Could you check a few things on this model? Use its own coordinates, in mm. A direction names the side the tool comes from. Give positions to 0.01 mm unless a question says otherwise; leave off trailing zeros. Write each loop counter-clockwise with the first axis right and the second up, starting at its lowest first coordinate (ties: lowest second). Pieces come first, ordered by that corner, then holes. Notation, with made-up numbers: M 64,5.25 L 89,5.25 A16 ccw 89,14.25 Z; hole C 53,72.25 d5. An arc over 180 degrees is marked long. Use one line per item in the form item = value.
from build123d import *

# Parameters (mm, degrees)
SKETCH1_R                             = 6
SKETCH1_R_2                           = 1.5
DISPLAY_SCREW_PATTERN_DEPTH           = 3
DISPLAY_SCREW_PATTERN_2_DEPTH         = 3
DISPLAY_SCREW_PATTERN_3_DEPTH         = 3
DISPLAY_SCREW_PATTERN_4_DEPTH         = 3
DISPLAY_SCREW_PATTERN_5_DEPTH         = 3
SKETCH2_W                             = 311.1
SKETCH2_H                             = 132.6
SKETCH2_R                             = 4
DISPLAY_BACKPLANE_DEPTH               = 3
BACKPLANE_WEIGHT_REDUCTION_DEPTH      = 203.770122306
BACKPLANE_WEIGHT_REDUCTION_DEPTH_BACK = 203.770122306
SKETCH4_W                             = 311.1
SKETCH4_H                             = 132.6
SKETCH4_W_2                           = 309.1
SKETCH4_H_2                           = 130.6
DISPLAY_OUTSIDE_CRADDLE_DEPTH         = 12
BOTTOM_RADIO_MOUNT_TABS_DEPTH         = 5
TOP_RADIO_MOUNT_TABS_DEPTH            = 5
TOP_RADIO_MOUNT_TABS_2_DEPTH          = 5
BOSS_EXTRUDE6_REACH                   = 208.065
BOSS_EXTRUDE7_REACH                   = 211.446
BOSS_EXTRUDE8_REACH                   = 213.846
BOSS_EXTRUDE9_REACH                   = 205.9
TAB_FILLETS_10MM_R                    = 10


with BuildPart() as part:
    # Sketch1 → Display screw pattern (new body)
    with BuildSketch(Plane.XY):
        Circle(SKETCH1_R)
        Circle(SKETCH1_R_2, mode=Mode.SUBTRACT)
    extrude(amount=DISPLAY_SCREW_PATTERN_DEPTH)



with BuildPart() as body_2:
    # Sketch1 → Display screw pattern 2 (new body)
    with BuildSketch(Plane.XY):
        with Locations((-106.24, 18.83)):
            Circle(SKETCH1_R)
        with Locations((-106.24, 18.83)):
            Circle(SKETCH1_R_2, mode=Mode.SUBTRACT)
    extrude(amount=DISPLAY_SCREW_PATTERN_2_DEPTH)


with BuildPart() as body_3:
    # Sketch1 → Display screw pattern 3 (new body)
    with BuildSketch(Plane.XY):
        with Locations((147.61, 18.83)):
            Circle(SKETCH1_R)
        with Locations((147.61, 18.83)):
            Circle(SKETCH1_R_2, mode=Mode.SUBTRACT)
    extrude(amount=DISPLAY_SCREW_PATTERN_3_DEPTH)


with BuildPart() as body_4:
    # Sketch1 → Display screw pattern 4 (new body)
    with BuildSketch(Plane.XY):
        with Locations((-121.24, -91.25)):
            Circle(SKETCH1_R)
        with Locations((-121.24, -91.25)):
            Circle(SKETCH1_R_2, mode=Mode.SUBTRACT)
    extrude(amount=DISPLAY_SCREW_PATTERN_4_DEPTH)


with BuildPart() as body_5:
    # Sketch1 → Display screw pattern 5 (new body)
    with BuildSketch(Plane.XY):
        with Locations((162.61, -91.25)):
            Circle(SKETCH1_R)
        with Locations((162.61, -91.25)):
            Circle(SKETCH1_R_2, mode=Mode.SUBTRACT)
    extrude(amount=DISPLAY_SCREW_PATTERN_5_DEPTH)


with BuildPart() as part_1:
    add(part.part)

    add(body_2.part)  # Display backplane merges body 2

    add(body_3.part)  # Display backplane merges body 3

    add(body_4.part)  # Display backplane merges body 4

    add(body_5.part)  # Display backplane merges body 5
    # Sketch2 → Display backplane (add)
    with BuildSketch(Plane(origin=(0, 0, 0), x_dir=(-1, 0, 0), z_dir=(0, 0, -1))):
        with Locations((-20.21, -34.77)):
            Rectangle(SKETCH2_W, SKETCH2_H)
        with Locations((106.24, 18.83)):
            Circle(SKETCH2_R, mode=Mode.SUBTRACT)
        Circle(SKETCH2_R, mode=Mode.SUBTRACT)
        with Locations((121.24, -91.25)):
            Circle(SKETCH2_R, mode=Mode.SUBTRACT)
        with Locations((-147.61, 18.83)):
            Circle(SKETCH2_R, mode=Mode.SUBTRACT)
        with Locations((-162.61, -91.25)):
            Circle(SKETCH2_R, mode=Mode.SUBTRACT)
    extrude(amount=DISPLAY_BACKPLANE_DEPTH)

    # Sketch3 → Backplane weight reduction (cut, two sides: drawn at the far end of the back side and taken through both)
    with BuildSketch(Plane.XY.offset(-BACKPLANE_WEIGHT_REDUCTION_DEPTH_BACK)):
        with BuildLine():
            Line((162.61, -7.17), (162.61, -67.25))
            ThreePointArc((162.61, -67.25), (160.930502943, -72.797001962), (156.456153846, -76.480769231))
            ThreePointArc((156.456153846, -76.480769231), (151.296291501, -79.936291501), (147.840769231, -85.096153846))
            ThreePointArc((147.840769231, -85.096153846), (144.157001962, -89.570502943), (138.61, -91.25))
            Line((138.61, -91.25), (-97.24, -91.25))
            ThreePointArc((-97.24, -91.25), (-102.787001962, -89.570502943), (-106.470769231, -85.096153846))
            ThreePointArc((-106.470769231, -85.096153846), (-109.926291501, -79.936291501), (-115.086153846, -76.480769231))
            ThreePointArc((-115.086153846, -76.480769231), (-119.560502943, -72.797001962), (-121.24, -67.25))
            Line((-121.24, -67.25), (-121.24, -7.17))
            ThreePointArc((-121.24, -7.17), (-118.311067812, -0.098932188), (-111.24, 2.83))
            Line((-111.24, 2.83), (-106.24, 2.83))
            ThreePointArc((-106.24, 2.83), (-97.36479686, 5.517195291), (-91.470769231, 12.676153846))
            ThreePointArc((-91.470769231, 12.676153846), (-87.787001962, 17.150502943), (-82.24, 18.83))
            Line((-82.24, 18.83), (-21, 18.83))
            ThreePointArc((-21, 18.83), (-13.928932188, 15.901067812), (-11, 8.83))
            Line((-11, 8.83), (-11, 0))
            ThreePointArc((-11, 0), (0, -11), (11, 0))
            Line((11, 0), (11, 8.83))
            ThreePointArc((11, 8.83), (13.928932188, 15.901067812), (21, 18.83))
            Line((21, 18.83), (123.61, 18.83))
            ThreePointArc((123.61, 18.83), (129.157001962, 17.150502943), (132.840769231, 12.676153846))
            ThreePointArc((132.840769231, 12.676153846), (138.73479686, 5.517195291), (147.61, 2.83))
            Line((147.61, 2.83), (152.61, 2.83))
            ThreePointArc((152.61, 2.83), (159.681067812, -0.098932188), (162.61, -7.17))
        make_face()
    extrude(amount=BACKPLANE_WEIGHT_REDUCTION_DEPTH + BACKPLANE_WEIGHT_REDUCTION_DEPTH_BACK, mode=Mode.SUBTRACT)

    # Sketch4 → Display outside craddle (add)
    with BuildSketch(Plane(origin=(0, 0, -3), x_dir=(-1, 0, 0), z_dir=(0, 0, -1))):
        with Locations((-20.21, -34.77)):
            Rectangle(SKETCH4_W, SKETCH4_H)
        with Locations((-20.21, -34.77)):
            Rectangle(SKETCH4_W_2, SKETCH4_H_2, mode=Mode.SUBTRACT)
    extrude(amount=DISPLAY_OUTSIDE_CRADDLE_DEPTH)

    # Sketch9 → Boss-Extrude6 (add, up to next)
    with BuildSketch(Plane(origin=(0, -9.845, 0), x_dir=(1, 0, 0), z_dir=(0, 1, 0)), mode=Mode.PRIVATE) as boss_extrude6_sk1:
        Polygon((109.074247912, 3), (134.956152423, 3), (135.76, 0), (109.87809549, 0), align=None)
    boss_extrude6_tool1 = extrude(boss_extrude6_sk1.sketch, amount=BOSS_EXTRUDE6_REACH, mode=Mode.PRIVATE) - part_1.part
    # Sketch9 → Boss-Extrude6 (add, up to next)
    with BuildSketch(Plane(origin=(0, -9.845, 0), x_dir=(1, 0, 0), z_dir=(0, 1, 0)), mode=Mode.PRIVATE) as boss_extrude6_sk2:
        Polygon((-58.122855224, 3), (-32.240950714, 3), (-31.437103136, 0), (-57.319007646, 0), align=None)
    boss_extrude6_tool2 = extrude(boss_extrude6_sk2.sketch, amount=BOSS_EXTRUDE6_REACH, mode=Mode.PRIVATE) - part_1.part


with BuildPart() as body_2_2:
    # Sketch5 → Bottom radio mount tabs (new body)
    with BuildSketch(Plane(origin=(0, -72.095, 0), x_dir=(1, 0, 0), z_dir=(0, 1, 0))):
        with BuildLine():
            Line((134.956152423, 3), (147.909153247, -45.341257188))
            ThreePointArc((147.909153247, -45.341257188), (147.20985029, -50.652990504), (142.959405779, -53.914471288))
            Line((142.959405779, -53.914471288), (132.33422169, -56.761480784))
            ThreePointArc((132.33422169, -56.761480784), (127.022488374, -56.062177826), (123.76100759, -51.811733316))
            Line((123.76100759, -51.811733316), (109.074247912, 3))
            Line((109.074247912, 3), (134.956152423, 3))
        make_face()
    extrude(amount=BOTTOM_RADIO_MOUNT_TABS_DEPTH)


with BuildPart() as body_3_2:
    # Sketch7 → Top radio mount tabs (new body)
    with BuildSketch(Plane(origin=(0, -14.845, 0), x_dir=(1, 0, 0), z_dir=(0, 1, 0))):
        with BuildLine():
            Line((-32.240950714, 3), (-19.287949889, -45.341257188))
            ThreePointArc((-19.287949889, -45.341257188), (-19.987252846, -50.652990504), (-24.237697357, -53.914471288))
            Line((-24.237697357, -53.914471288), (-34.862881446, -56.761480784))
            ThreePointArc((-34.862881446, -56.761480784), (-40.174614762, -56.062177826), (-43.436095546, -51.811733316))
            Line((-43.436095546, -51.811733316), (-58.122855224, 3))
            Line((-58.122855224, 3), (-32.240950714, 3))
        make_face()
    extrude(amount=TOP_RADIO_MOUNT_TABS_DEPTH)


with BuildPart() as body_4_2:
    # Sketch7 → Top radio mount tabs 2 (new body)
    with BuildSketch(Plane(origin=(0, -14.845, 0), x_dir=(1, 0, 0), z_dir=(0, 1, 0))):
        with BuildLine():
            Line((132.33422169, -56.761480784), (142.959405779, -53.914471288))
            ThreePointArc((142.959405779, -53.914471288), (147.20985029, -50.652990504), (147.909153247, -45.341257188))
            Line((147.909153247, -45.341257188), (134.956152423, 3))
            Line((134.956152423, 3), (109.074247912, 3))
            Line((109.074247912, 3), (123.76100759, -51.811733316))
            ThreePointArc((123.76100759, -51.811733316), (127.022488374, -56.062177826), (132.33422169, -56.761480784))
        make_face()
    extrude(amount=TOP_RADIO_MOUNT_TABS_2_DEPTH)


with BuildPart() as part_2:
    add(part_1.part)

    add(body_3_2.part)  # Boss-Extrude6 merges body 3 2

    add(body_4_2.part)  # Boss-Extrude6 merges body 4 2
    add(boss_extrude6_tool1.solids().sort_by_distance((122.417124, -9.845, -1.5))[0])
    add(boss_extrude6_tool2.solids().sort_by_distance((-44.779979, -9.845, -1.5))[0])

    # Sketch10 → Boss-Extrude7 (add, up to next)
    with BuildSketch(Plane(origin=(0, -67.095, 0), x_dir=(1, 0, 0), z_dir=(0, 1, 0)), mode=Mode.PRIVATE) as boss_extrude7_sk1:
        Polygon((109.074247912, 3), (109.87809549, 0), (135.76, 0), (134.956152423, 3), align=None)
    boss_extrude7_tool1 = extrude(boss_extrude7_sk1.sketch, amount=BOSS_EXTRUDE7_REACH, mode=Mode.PRIVATE) - part_2.part

    add(body_2_2.part)  # Boss-Extrude7 merges body 2 2
    add(boss_extrude7_tool1.solids().sort_by_distance((122.417124, -67.095, -1.5))[0])

    # Sketch11 → Boss-Extrude8 (add, up to next)
    with BuildSketch(Plane.XZ.offset(72.095), mode=Mode.PRIVATE) as boss_extrude8_sk1:
        Polygon((134.956152423, -3), (109.074247912, -3), (109.87809549, 0), (135.76, 0), align=None)
    boss_extrude8_tool1 = extrude(boss_extrude8_sk1.sketch, amount=BOSS_EXTRUDE8_REACH, mode=Mode.PRIVATE) - part_2.part
    add(boss_extrude8_tool1.solids().sort_by_distance((122.417124, -72.095, -1.5))[0])

    # Sketch12 → Boss-Extrude9 (add, up to next)
    with BuildSketch(Plane.XZ.offset(14.845), mode=Mode.PRIVATE) as boss_extrude9_sk1:
        Polygon((-32.240950714, -3), (-58.122855224, -3), (-57.319007646, 0), (-31.437103136, 0), align=None)
    boss_extrude9_tool1 = extrude(boss_extrude9_sk1.sketch, amount=BOSS_EXTRUDE9_REACH, mode=Mode.PRIVATE) - part_2.part
    add(boss_extrude9_tool1.solids().sort_by_distance((-44.779979, -14.845, -1.5))[0])

    # Tab fillets 10mm
    tab_fillets_10mm_edges = [part_2.edges().sort_by_distance(p)[0] for p in [
        (122.819047745, -9.845, 0),
        (-44.378055391, -9.845, 0),
        (122.819047745, -14.845, 0),
        (122.819047745, -67.095, 0),
        (122.819047745, -72.095, 0),
        (-44.378055391, -14.845, 0),
    ]]
    fillet(tab_fillets_10mm_edges, radius=TAB_FILLETS_10MM_R)


solid = part_2.part
1) I want a section at D-D, the plane x = 18. Please give me the cut outline in (y, z).
Checked values:
outline = M -101.07,-15 L -100.07,-15 L -100.07,-3 L -91.25,-3 L -91.25,0 L -101.07,0 Z; M 18.37,-3 L 30.53,-3 L 30.53,-15 L 31.53,-15 L 31.53,0 L 18.37,0 Z
2) Thinking about a two-plate mould opening in Y: for faces 6 (the flat face through (22, -100.07, -9)), 7 (the flat face through (131, -72.095, 33)), 8 (the cylindrical face through (123.959, -6.838, 2.852)), which applies, released by +Y, released by -Y, zero draft, split by the parting line, or undercut?
Checked values:
face_6 = undercut
face_7 = released by -Y
face_8 = released by +Y
3) I want a section at A-A, the plane x = -61.5. Please give me the cut outline in (y, z).
Checked values:
outline = M -101.07,-15 L -100.07,-15 L -100.07,-3 L -91.25,-3 L -91.25,0 L -101.07,0 Z; M 18.83,-3 L 30.53,-3 L 30.53,-15 L 31.53,-15 L 31.53,0 L 18.83,0 Z
4) If I drill on L1, parallel to Y at x = -106.24, z = -1.95; L2, parallel to Y at x = -40.5, z = -11.5; L3, parallel to Z at x = -50.5, y = 3, over which ranges is the centre line in solid material (lowest first)?
Checked values:
L1 = -101.07 to -85.61, 2.83 to 14.83, 22.83 to 31.53
L2 = -101.07 to -100.07, 30.53 to 31.53
L3 = -3 to 0
5) I want a section at C-C, the plane y = -18. Please give me the cut outline in (x, z), plus the area to 3 significant figures.
Checked values:
outline = M -135.34,-15 L -134.34,-15 L -134.34,-3 L -121.24,-3 L -121.24,0 L -135.34,0 Z; M -58.12,-3 L -32.24,-3 L -30.71,2.71 L -56.59,2.71 Z; M 109.07,-3 L 134.96,-3 L 136.49,2.71 L 110.6,2.71 Z; M 162.61,-3 L 174.76,-3 L 174.76,-15 L 175.76,-15 L 175.76,0 L 162.61,0 Z
area = 401 mm2
6) I want a section at B-B, the plane z = 23. Please give me the cut outline in (x, y) (3 decimals).
Checked values:
outline = M -51.156,-14.845 L -25.274,-14.845 L -25.274,-9.845 L -51.156,-9.845 Z; M 116.041,-72.095 L 141.923,-72.095 L 141.923,-67.095 L 116.041,-67.095 Z; M 116.041,-14.845 L 141.923,-14.845 L 141.923,-9.845 L 116.041,-9.845 Z
7) For faces 1 (the cylindrical face through (-40.11, -12.38, 56.1)), 2 (the cylindrical face through (148.477, 14.925, -1.479)), 3 (the cylindrical face through (-42.838, -17.852, 2.852)), 4 (the cylindrical face through (168.333, -89.448, 1.479)), 5 (the cylindrical face through (-109.865, -79.998, -1.521)), which set-ups out of +Z, -Z, +X, -X, +Y, -Y let a thin tool reach every point of the face, with its end or its side?
Checked values:
face_1 = +Z, +Y, -Y
face_2 = -Z
face_3 = +Z, +X, -X, -Y
face_4 = +Z
face_5 = +Z, -Z
8) For pin 1 Ø13 at (x, y) = (0, 0) entering from -Z; pin 2 Ø18 at (x, z) = (-37.5, 37) entering from -Y (3 decimals); pin 3 Ø2 at (x, y) = (110, -43) entering from +Z, each with a flat end and sliding along its axis, tell me the tip position at first contact or that it passes through.
Checked values:
pin_1 = -3
pin_2 = -14.845
pin_3 = 0
